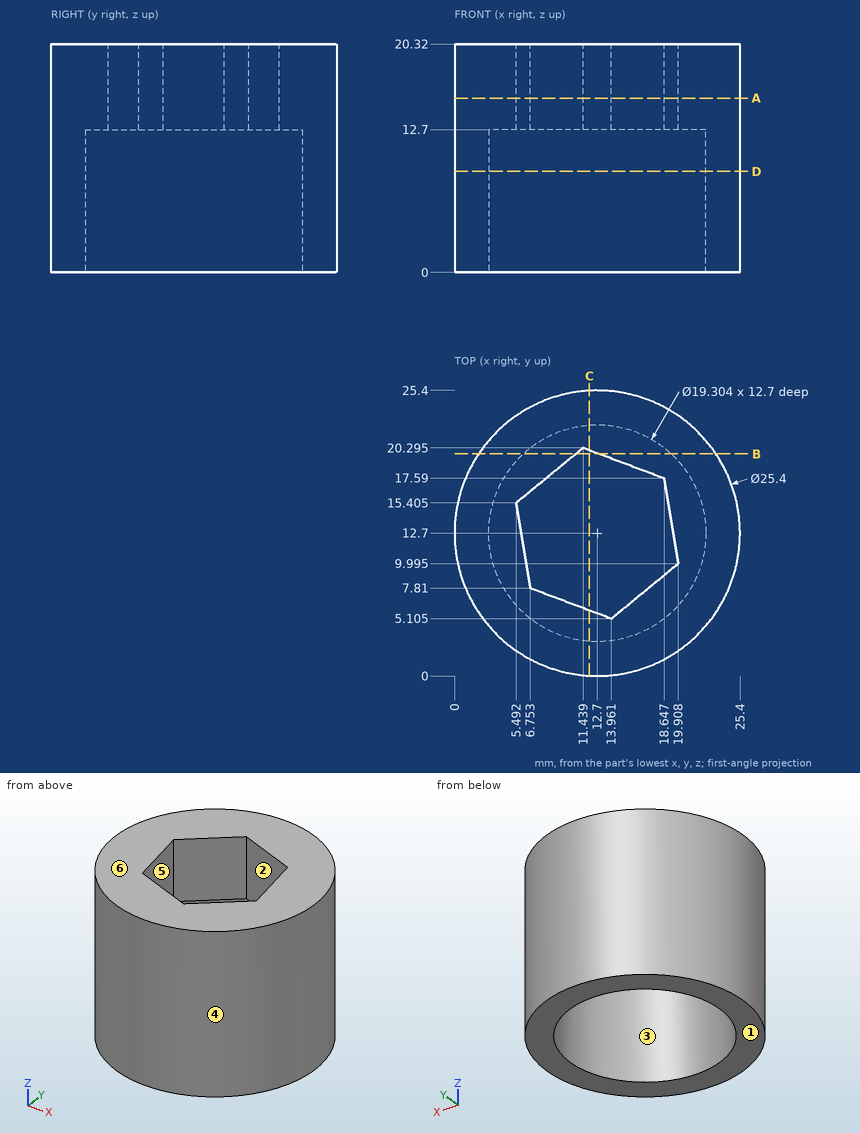
Study the drawing (mm; zero at the part's minimum x, y, z) and answer. A direction names the side the tool comes from. Coordinates: 2 decimals unless noted, no trailing zeros. Loops run counter-clockwise (first coordinate to the right, second up) from the corner with the lowest first, then second, coordinate; pieces in that order, holes last. Notation, with made-up numbers: M 69,27 L 83,27 A29 ccw 83,49 Z; hole C 24.5,77 d1. An arc over 180 degrees is marked long. Answer in a Markdown table with one row per item.
1) Find section D-D (z = 9). Determine the outline of the cut face in (x, y), then the cut area to 3 significant figures.
Answers below:
| item | result |
|---|---|
| outline | C 12.7,12.7 d25.4; hole C 12.7,12.7 d19.3 |
| area | 214 mm^2 |
2) Find section C-C (x = 12). Determine the outline of the cut face in (y, z) (1 decimal), then the cut area to 3 significant figures.
Answers below:
| item | result |
|---|---|
| outline | M 0,0 L 3.1,0 L 3.1,12.7 L 5.8,12.7 L 5.8,20.3 L 0,20.3 Z; M 20.1,12.7 L 22.3,12.7 L 22.3,0 L 25.4,0 L 25.4,20.3 L 20.1,20.3 Z |
| area | 162 mm^2 |
3) Find section B-B (y = 19.75). Determine the outline of the cut face in (x, z).
Answers below:
| item | result |
|---|---|
| outline | M 2.14,0 L 6.11,0 L 6.11,12.7 L 10.78,12.7 L 10.78,20.32 L 2.14,20.32 Z; M 12.89,12.7 L 19.29,12.7 L 19.29,0 L 23.26,0 L 23.26,20.32 L 12.89,20.32 Z |
4) Find section A-A (z = 15.5). Determine the outline of the cut face in (x, y) (1 decimal), then the cut area to 3 significant figures.
Answers below:
| item | result |
|---|---|
| outline | C 12.7,12.7 d25.4; hole M 5.5,15.4 L 6.8,7.8 L 14,5.1 L 19.9,10 L 18.6,17.6 L 11.4,20.3 Z |
| area | 353 mm^2 |
5) Which of the six approach directions +Z, -Z, +X, -X, +Y, -Y give full straight-line access (tool end or side, diameter ignored) to the marked faces 1, 2 and 3?
Answers below:
| item | result |
|---|---|
| face 1 | -Z, +X, -X, +Y, -Y |
| face 2 | +Z, -Z |
| face 3 | -Z |
6) Determine the mould class of the marked faces 4, 5 and 6 for opening direction X: released by +X, released by -X, zero draft, split by the parting line, or undercut.
Answers below:
| item | result |
|---|---|
| face 4 | split by the parting line |
| face 5 | undercut |
| face 6 | zero draft |
7) Find the intervals of material crossed by probe 1 along Y at (x, z) = (11, 3.75) (1 decimal); probe 2 along Y at (x, z) = (19, 12); probe 3 along X at (y, z) = (13.25, 13), in increasing order.
Answers below:
| item | result |
|---|---|
| probe 1 | 0.1 to 3.2, 22.2 to 25.3 |
| probe 2 | 1.67 to 5.39, 20.01 to 23.73 |
| probe 3 | 0.01 to 5.85, 19.37 to 25.39 |
8) Given pin 1 (5 mm diameter, centred on x = 17.5, z = 18, fed in from -Y); pin 2 (1 mm diameter, centred on y = 11, z = 13.5, fed in from +X); pin 3 (5 mm diameter, centred on y = 4.5, z = 12.5, fed in from +X); pin 4 (11.5 mm diameter, centred on x = 12.7, y = 12.7, fed in from +Z), each flat-ended and moving along its own axis, determine where each tip first touches the part or whether it passes through.
Answers below:
| item | result |
|---|---|
| pin 1 | y = 0.21 |
| pin 2 | x = 25.34 |
| pin 3 | x = 24.05 |
| pin 4 | through |
